Part model, mm, in its own coordinate system. A direction names the side the tool comes from. Coordinates: 2 decimals unless noted, no trailing zeros. Loops run counter-clockwise (first coordinate to the right, second up) from the corner with the lowest first, then second, coordinate; pieces in that order, holes last. Notation, with made-up numbers: (-6, -4.5) -> (17, -4.5) arc R13 ccw to (17, 8.5) -> close; hole circle Ø6 at (44.5, 69.25). An arc over 180 degrees is marked (long way). One line per item, written item: value. Start each with the question number.
from build123d import *

# Parameters (mm, degrees)
SKETCH3_W           = 120
SKETCH3_H           = 120
BOSS_EXTRUDE2_DEPTH = 50
SKETCH4_R           = 35
BOSS_EXTRUDE3_DEPTH = 45
SKETCH9_R           = 25
CUT_EXTRUDE3_DEPTH  = 195.486503388
FILLET4_R           = 10
FILLET5_R           = 1.5
SHELL2_T            = -2


with BuildPart() as part:
    # Sketch3 → Boss-Extrude2 (new body)
    with BuildSketch(Plane(origin=(0, 0, 0), x_dir=(1, 0, 0), z_dir=(0, 1, 0))):
        with Locations((60, 60)):
            Rectangle(SKETCH3_W, SKETCH3_H)
    extrude(amount=BOSS_EXTRUDE2_DEPTH)

    # Sketch4 → Boss-Extrude3 (add)
    with BuildSketch(Plane(origin=(0, 50, 0), x_dir=(1, 0, 0), z_dir=(0, 1, 0))):
        with Locations(Location((60, 60, 0), (0, 0, 90))):
            Circle(SKETCH4_R)
    extrude(amount=BOSS_EXTRUDE3_DEPTH)

    # Sketch9 → Cut-Extrude3 (cut, through all)
    with BuildSketch(Plane(origin=(0, 95, 0), x_dir=(1, 0, 0), z_dir=(0, 1, 0))):
        with Locations(Location((60, 60, 0), (0, 0, 270))):
            Circle(SKETCH9_R)
    extrude(amount=-CUT_EXTRUDE3_DEPTH, mode=Mode.SUBTRACT)

    # Fillet4
    fillet4_edges = [part.edges().sort_by_distance(p)[0] for p in [
        (60, 50, 0),
        (60, 50, -25),
        (0, 50, -60),
        (60, 50, -120),
        (0, 25, -120),
        (0, 25, 0),
        (120, 25, 0),
        (120, 25, -120),
        (120, 50, -60),
    ]]
    fillet(fillet4_edges, radius=FILLET4_R)

    # Fillet5
    fillet5_edges = [part.edges().sort_by_distance(p)[0] for p in [
        (60, 95, -25),
        (60, 95, -85),
    ]]
    fillet(fillet5_edges, radius=FILLET5_R)

    # Shell2
    shell2_openings = [part.faces().sort_by_distance(p)[0] for p in [
        (60, 0, -1.697056275),
    ]]
    offset(amount=SHELL2_T, openings=shell2_openings, kind=Kind.INTERSECTION)


solid = part.part
1) Pull direction Z, two halves, no side cores. Call faces 4 (the cylindrical face through (2.85, 20.28, -3.01)), 5 (the flat face through (120, 20, -59)), 6 (the cylindrical face through (115.594, 45.719, -60.7)): +Z half, -Z half, draft (parallel to the pull), parting line (faces both ways), or undercut.
2) Pin check, flat tips, straight feed: pin 1 Ø1 at (x, y) = (42, 73.5) entering from -Z; pin 2 Ø12 at (x, z) = (66.5, -95.5) entering from -Y; pin 3 Ø3 at (y, z) = (60, -43) entering from -X. Stop position of each tip, or through.
3) Tool access for faces 1 (the cylindrical face through (2.85, 20.28, -116.99)), 2 (the cylindrical face through (25.3, 76.52, -55.44)), 3 (the cylindrical face through (4.281, 20.28, -115.594)): list every direction of +Z, -Z, +X, -X, +Y, -Y with a clear straight run to the whole face (end or side of a thin tool).
4) Slice it at B-B (y = 69). Give the cut face in (x, z), then the cut area to 3 significant figures.
5) Slice it at A-A (y = 14). Give the cut face in (x, z).
6) Probe line 1 (X direction, y = 73, z = -60); line 2 (Z direction, x = 66, y = 12.5); line 3 (Z direction, x = 58.5, y = 80.5). List the from-to ranges inside material, lowest first. Write a range as from..to.
Check sheet entries:
1. face 4: +Z half
1. face 5: draft
1. face 6: undercut
2. pin 1: stops at z = -90.31
2. pin 2: stops at y = 48.36
2. pin 3: stops at x = 28.62
3. face 1: -Z, -X, +Y, -Y
3. face 2: +Y
3. face 3: -Y
4. outline: circle Ø70 at (60, -60); circle Ø54 at (60, -60); hole circle Ø66 at (60, -60); hole circle Ø50 at (60, -60)
4. area: 754 mm^2
5. outline: (0, -110) arc R10 ccw to (10, -120) -> (110, -120) arc R10 ccw to (120, -110) -> (120, -10) arc R10 ccw to (110, 0) -> (10, 0) arc R10 ccw to (0, -10) -> close; circle Ø54 at (60, -60); hole (2, -110) arc R8 ccw to (10, -118) -> (110, -118) arc R8 ccw to (118, -110) -> (118, -10) arc R8 ccw to (110, -2) -> (10, -2) arc R8 ccw to (2, -10) -> close; hole circle Ø50 at (60, -60)
6. line 1: x = 25..27, 33..35, 85..87, 93..95
6. line 2: z = -120..-118, -86.32..-84.27, -35.73..-33.68, -2..0
6. line 3: z = -94.97..-92.97, -86.96..-84.95, -35.05..-33.04, -27.03..-25.03
